```python
from build123d import *

# Parameters (mm, degrees)
BOSS_EXTRUDE1_DEPTH = 160
CUT_EXTRUDE1_DEPTH  = 150


with BuildPart() as part:
    # Sketch1 → Boss-Extrude1 (new body)
    with BuildSketch(Plane(origin=(0, 0, 0), x_dir=(1, 0, 0), z_dir=(0, 1, 0))):
        with BuildLine():
            Line((-40, 91.651513899), (-40, 80))
            Line((-40, 80), (40, 80))
            Line((40, 80), (40, 91.651513899))
            ThreePointArc((40, 91.651513899), (0, -100), (-40, 91.651513899))
        make_face()
    extrude(amount=-BOSS_EXTRUDE1_DEPTH)

    # Sketch2 → Cut-Extrude1 (cut)
    with BuildSketch(Plane(origin=(0, 0, 0), x_dir=(1, 0, 0), z_dir=(0, 1, 0))):
        with BuildLine():
            Line((50, 70), (-50, 70))
            Line((-50, 70), (-56.568542495, 70))
            ThreePointArc((-56.568542495, 70), (0, -90), (56.568542495, 70))
            Line((56.568542495, 70), (50, 70))
        make_face()
    extrude(amount=-CUT_EXTRUDE1_DEPTH, mode=Mode.SUBTRACT)


solid = part.part
```
Input: part model. Units: mm. Frame: model coordinates. A direction names the side the tool comes from. Coordinates: 2 decimals unless noted, no trailing zeros. Write each loop counter-clockwise with the first axis right and the second up, starting at its lowest first coordinate (ties: lowest second). Pieces come first, ordered by that corner, then holes. Notation, with made-up numbers: (-38.5, 32) - (-13.5, 32) arc R10 cw to (-13.5, 50) - close; hole circle Ø6 at (-9.5, 11). An arc over 180 degrees is marked (long way). Put each result on its own line as item: value. Start each with the question number.
1) Ray query, L1, parallel to Z at x = 0, y = -98.5; L2, parallel to X at y = -30.5, z = 0; L3, parallel to Y at x = 47, z = 16. Return the intervals inside material, ascending.
2) Cut plane A-A (y = -44.5). Return the cut outline in (x, z).
3) Mould query, pull axis X, two halves, no side actions, for faces 1 (the face through (-3.101, -73.95, 89.947)), 2 (the face through (3.821, -78.88, 99.927)), 3 (the face through (0, 0, -74)), 4 (the face through (-40, -79, -86)). Classes: pulls with the +X half, pulls with the -X half, needs draft (parallel to the pull), parting line crosses it, or undercut.
4) Contact query for flat-ended pins moving along their axis: pin 1 (5 mm diameter, centred on y = -36.5, z = 66.5, fed in from -X); pin 2 (2 mm diameter, centred on x = -24, y = -136, fed in from -Z); pin 3 (6 mm diameter, centred on y = -86.5, z = -83.5, fed in from -X). Output: stop coordinate, or through.
5) Cut plane B-B (x = 0). Return the cut outline in (y, z), plus the area to 3 significant figures.
6) Cut plane C-C (z = 0). Return the cut outline in (x, y), plus the area to 3 significant figures.
7) Reachability of faces 5 (the face through (1, -74, -70)), 6 (the face through (1, -160, 3)), 7 (the face through (40, -79, -86)) from +Z, -Z, +X, -X, +Y, -Y: full face, straight path, thin tool, end or side. Return the list, or none.
Resolved:
1. L1: z = -80 to -70, 90 to 100
1. L2: x = -100 to -90, 90 to 100
1. L3: y = -160 to -150
2. outline: (-40, -91.65) - (-40, -80) - (40, -80) - (40, -91.65) arc R100 ccw (long way) to start; hole (-56.57, -70) - (56.57, -70) arc R90 ccw (long way) to start
3. face 1: undercut
3. face 2: parting line crosses it
3. face 3: needs draft
3. face 4: undercut
4. pin 1: stops at x = -76.84
4. pin 2: stops at z = -80
4. pin 3: stops at x = -59.33
5. outline: (-160, -80) - (0, -80) - (0, -70) - (-150, -70) - (-150, 90) - (0, 90) - (0, 100) - (-160, 100) - close
5. area: 4,800 mm2
6. outline: (-100, -160) - (100, -160) - (100, 0) - (90, 0) - (90, -150) - (-90, -150) - (-90, 0) - (-100, 0) - close
6. area: 5,000 mm2
7. face 5: +Y
7. face 6: +Z, -Z, +X, -X, -Y
7. face 7: -Z, +Y, -Y
